Geometry check sheet. Reference: the model listing, model coordinates, mm. A direction names the side the tool comes from. Give positions to 0.01 mm unless a question says otherwise; leave off trailing zeros. Loops run counter-clockwise (first coordinate to the right, second up) from the corner with the lowest first, then second, coordinate; pieces in that order, holes last.
```python
from build123d import *

# Parameters (mm, degrees)
SKETCH_1_W                   = 50
SKETCH_1_H                   = 5.1
EXTRUDE_1_DEPTH              = 4
SKETCH_3_W                   = 50
SKETCH_3_H                   = 25
EXTRUDE_2_DEPTH              = 10
SKETCH_4_W                   = 10
SKETCH_4_H                   = 25
EXTRUDE_3_DEPTH              = 50
SKETCH_5_W                   = 150
SKETCH_5_H                   = 30
EXTRUDE_4_DEPTH              = 10
CUT_EXTRUDE_START            = -20
SKETCH_6_W                   = 150
SKETCH_6_H                   = 0.8
CUT_EXTRUDE_1_DEPTH          = 20
HOLE_WIZARD_M4_1_D           = 4.3
HOLE_WIZARD_M4_1_CBORE_D     = 8
HOLE_WIZARD_M4_1_CBORE_DEPTH = 4


with BuildPart() as part:
    # 스케치1 → 보스-돌출1 (new body)
    with BuildSketch(Plane.XY):
        Rectangle(SKETCH_1_W, SKETCH_1_H)
    extrude(amount=EXTRUDE_1_DEPTH)

    # 스케치3 → 보스-돌출2 (add)
    with BuildSketch(Plane.XY.offset(4)):
        with Locations((0, -2.5)):
            Rectangle(SKETCH_3_W, SKETCH_3_H)
    extrude(amount=EXTRUDE_2_DEPTH)

    # 스케치4 → 보스-돌출3 (add)
    with BuildSketch(Plane.ZY.offset(25)):
        with Locations((9, -2.5)):
            Rectangle(SKETCH_4_W, SKETCH_4_H)
    extrude_3 = extrude(amount=EXTRUDE_3_DEPTH)

    # 대칭 복사1: 보스-돌출3 across plane
    add(extrude_3.mirror(Plane.ZY))

    # 스케치5 → 보스-돌출4 (add)
    with BuildSketch(Plane.XZ.offset(15)):
        with Locations((0, -1)):
            Rectangle(SKETCH_5_W, SKETCH_5_H)
    extrude(amount=EXTRUDE_4_DEPTH)

    # 스케치6 → 컷-돌출1 (cut)
    with BuildSketch(Plane(origin=(0, 0, -16), x_dir=(-1, 0, 0), z_dir=(0, 0, -1)).offset(CUT_EXTRUDE_START)):
        with Locations((0, -15.4)):
            Rectangle(SKETCH_6_W, SKETCH_6_H)
    extrude(amount=CUT_EXTRUDE_1_DEPTH, mode=Mode.SUBTRACT)

    # M4 소켓 머리 캡 나사용 카운터보어1 (through all)
    with Locations(Plane.XY.offset(14)):
        with Locations((-65, 0), (65, 0)):
            CounterBoreHole(HOLE_WIZARD_M4_1_D / 2, HOLE_WIZARD_M4_1_CBORE_D / 2, HOLE_WIZARD_M4_1_CBORE_DEPTH)


solid = part.part
```
1) Depth check by flat-ended pin: P1, Ø5.5, axis at x = -11, y = -0.5, coming from the -Z side; P2, Ø5, axis at x = -65, y = 0, coming from the +Z side; P3, Ø9, axis at x = -64, y = 1, coming from the +Z side; P4, Ø2, axis at x = 1, z = 2, coming from the +Y side. Enter the tip coordinate at first touch or a pass-through.
2) Sectioned sample at D-D on z = -10. Enter the section's corners in (x, y), plus the area to 3 significant figures.
3) Tool access check on faces 1 (the flat face through (-25, 0, 2)), 2 (the flat face through (67, -2, 10)), 3 (the flat face through (0, -2.55, 2)), 4 (the flat face through (0, 2.55, 2)), 5 (the flat face through (25, 0, 2)). Record the directions out of +Z, -Z, +X, -X, +Y, -Y that give a thin tool (end or side, any length) a straight path to the whole face; none if there is none.
4) Sectioned sample at B-B on x = -65. Enter the section's corners in (y, z), plus the area to 3 significant figures.
5) Scan lines: line 1 along Y through (x, z) = (-65, 13.15); line 2 along Y through (x, z) = (-15, 1.5); line 3 along Y through (x, z) = (50.5, 0.75). Record each from-to range of solid material in increasing order.
6) Mould release check, pull along X, two halves, no side actions. Record for faces 6 (the flat face through (-63, -2, 10)), 7 (the flat face through (1, -15.8, -6)), 8 (the flat face through (75, -11, 5)): +X half, -X half, draft (parallel to the pull), parting line (faces both ways), or undercut.
7) Sectioned sample at A-A on y = 0. Enter the section's corners in (x, z).
8) Sectioned sample at C-C on x = 5. Enter the section's corners in (y, z).
Determined:
1. P1: stops at z = 0
1. P2: stops at z = 10
1. P3: stops at z = 14
1. P4: stops at y = 2.55
2. outline: (-75, -25) - (75, -25) - (75, -15.8) - (-75, -15.8) - close
2. area: 1,380 mm2
3. face 1: -Z, -X, +Y
3. face 2: +Z
3. face 3: -Z, +X, -X
3. face 4: -Z, +X, -X, +Y
3. face 5: -Z, +X, +Y
4. outline: (-25, -16) - (-15.8, -16) - (-15.8, 4) - (-2.15, 4) - (-2.15, 10) - (-4, 10) - (-4, 14) - (-25, 14) - close; (2.15, 4) - (10, 4) - (10, 14) - (4, 14) - (4, 10) - (2.15, 10) - close
4. area: 476 mm2
5. line 1: y = -25 to -4, 4 to 10
5. line 2: y = -25 to -15.8, -2.55 to 2.55
5. line 3: y = -25 to -15.8
6. face 6: undercut
6. face 7: draft
6. face 8: +X half
7. outline: (-75, 4) - (-67.15, 4) - (-67.15, 10) - (-69, 10) - (-69, 14) - (-75, 14) - close; (-62.85, 4) - (-25, 4) - (-25, 0) - (25, 0) - (25, 4) - (62.85, 4) - (62.85, 10) - (61, 10) - (61, 14) - (-61, 14) - (-61, 10) - (-62.85, 10) - close; (67.15, 4) - (75, 4) - (75, 14) - (69, 14) - (69, 10) - (67.15, 10) - close
8. outline: (-25, -16) - (-15.8, -16) - (-15.8, 4) - (-2.55, 4) - (-2.55, 0) - (2.55, 0) - (2.55, 4) - (10, 4) - (10, 14) - (-25, 14) - close
